```python
from build123d import *

# Parameters (mm, degrees)
F0_R     = 63.5
F1_DEPTH = 152.4
F3_T     = -7.62


with BuildPart() as f1:
    # F0 (on Top) → F1 (new body)
    with BuildSketch(Plane.XY):
        with Locations((-8.565548, 9.538906)):
            Circle(F0_R)
    extrude(amount=F1_DEPTH)


with BuildPart() as f1_1:
    # F2: moved
    add(f1.part.moved(Location((8.56556, -9.53905, 0))))

    # F3
    f3_openings = [f1_1.faces().sort_by_distance(p)[0] for p in [
        (1.2e-05, -0.000144, 152.4),
    ]]
    offset(amount=F3_T, openings=f3_openings)


solid = f1_1.part
```
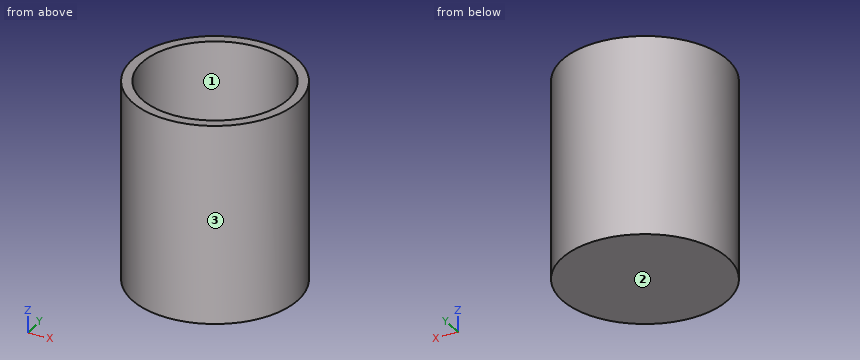
Could you check a few things on this model? Use its own coordinates, in mm. Face numbers are marked on the shaded views. Round coordinates to 2 decimals unless told otherwise and drop trailing zeros. Loops run counter-clockwise (first coordinate to the right, second up) from the corner with the lowest first, then second, coordinate; pieces in that order, holes last. Notation, with made-up numbers: M -6,78 L 9,78 A25 ccw 9,103 Z; hole C 7.5,-23 d2. An arc over 180 degrees is marked long. Put each result on its own line as item: value.
Q1. Imagine slicing it at C-C (z = 90). Write out the boundary of the cut face in (x, y), then the cut area to 3 significant figures.
Check result:
outline: C 0,0 d127; hole C 0,0 d111.76
area: 2,860 mm2
Q2. Thinking about a two-plate mould opening in Y: for the marked faces 1, 2 and 3, which applies, released by +Y, released by -Y, zero draft, split by the parting line, or undercut?
Check result:
face 1: undercut
face 2: zero draft
face 3: split by the parting line
Q3. Imagine slicing it at B-B (y = 16). Write out the boundary of the cut face in (x, z), then the cut area to 3 significant figures.
Check result:
outline: M -61.45,0 L 61.45,0 L 61.45,152.4 L 53.54,152.4 L 53.54,7.62 L -53.54,7.62 L -53.54,152.4 L -61.45,152.4 Z
area: 3,230 mm2
Q4. For pin 1 (1 mm diameter, centred on x = 34, z = 126, fed in from +Y); pin 2 (6 mm diameter, centred on x = 23, z = 35, fed in from -Y); pin 3 (1 mm diameter, centred on y = -14, z = 123.5, fed in from -X), each with a flat end and sliding along its axis, tell me the tip position at first contact or that it passes through.
Check result:
pin 1: y = 53.94
pin 2: y = -60.27
pin 3: x = -62.05
Q5. Imagine slicing it at A-A (x = 0). Write out the boundary of the cut face in (y, z).
Check result:
outline: M -63.5,0 L 63.5,0 L 63.5,152.4 L 55.88,152.4 L 55.88,7.62 L -55.88,7.62 L -55.88,152.4 L -63.5,152.4 Z
Q6. I need wall thicknesses on probe 1 along X at (y, z) = (0.5, 101.5); probe 2 along Z at (x, y) = (4, 10); probe 3 along X at (y, z) = (2, 68). Which ranges of each line are inside material? Lowest first, please.
Check result:
probe 1: -63.5 to -55.88, 55.88 to 63.5
probe 2: 0 to 7.62
probe 3: -63.47 to -55.84, 55.84 to 63.47
